Geometry check sheet. Reference: the model listing, model coordinates, mm. Give positions to 0.01 mm unless a question says otherwise; leave off trailing zeros. Loops run counter-clockwise (first coordinate to the right, second up) from the corner with the lowest first, then second, coordinate; pieces in that order, holes last.
1. Go/stop test with flat-tipped pins: pin 1 Ø1 at (y, z) = (-52, 1.5) entering from +X; pin 2 Ø3 at (y, z) = (-34, 9) entering from +X. Record where each tip stops, or that it passes through.
2. Cross-section at D-D, the plane y = -17. Record the cut outline in (x, z).
3. Cross-section at B-B, the plane x = -126.5. Record the cut outline in (y, z).
4. Release check for a two-part mould opening along Y. For faces 1 (the cylindrical face through (85.467, -33.361, 6.261)), 2 (the flat face through (-11, -32, 0)), 3 (the cylindrical face through (-153.58, -31.57, 6.26)) record: +Y half, -Y half, draft (parallel to the pull), parting line (faces both ways), or undercut.
5. Cross-section at A-A, the plane y = -28.5. Record the cut outline in (x, z).
6. Material ranges on L1, parallel to X at y = -32.5, z = 11.25; L2, parallel to X at y = -39, z = 11; L3, parallel to Y at x = -142.5, z = 6.5, recorded low to high.
from build123d import *

# Parameters (mm, degrees)
SKETCH1_R           = 20.32
BOSS_EXTRUDE1_DEPTH = 12.7


with BuildPart() as part:
    # Sketch1 → Boss-Extrude1 (new body)
    with BuildSketch(Plane.XY):
        with BuildLine():
            Line((37.409275597, 7.872494736), (-133.278879175, -7.060783805))
            ThreePointArc((-133.278879175, -7.060783805), (-158.678879175, -32.460783805), (-133.278879175, -57.860783805))
            Line((-133.278879175, -57.860783805), (37.409275597, -72.794062346))
            Line((37.409275597, -72.794062346), (44.521120825, -73.41626818))
            ThreePointArc((44.521120825, -73.41626818), (85.476605199, -32.460783805), (44.521120825, 8.49470057))
            Line((44.521120825, 8.49470057), (37.409275597, 7.872494736))
        make_face()
        with Locations((-133.278879175, -32.460783805)):
            Circle(SKETCH1_R, mode=Mode.SUBTRACT)
        with Locations((44.521120825, -32.460783805)):
            Circle(SKETCH1_R, mode=Mode.SUBTRACT)
    extrude(amount=BOSS_EXTRUDE1_DEPTH)


solid = part.part
Result:
1. pin 1: stops at x = 80.78
1. pin 2: stops at x = 85.48
2. outline: (-153.43, 0) - (-146.46, 0) - (-146.46, 12.7) - (-153.43, 12.7) - close; (-120.09, 0) - (31.34, 0) - (31.34, 12.7) - (-120.09, 12.7) - close; (57.71, 0) - (82.45, 0) - (82.45, 12.7) - (57.71, 12.7) - close
3. outline: (-58.45, 0) - (-51.62, 0) - (-51.62, 12.7) - (-58.45, 12.7) - close; (-13.3, 0) - (-6.47, 0) - (-6.47, 12.7) - (-13.3, 12.7) - close
4. face 1: parting line
4. face 2: draft
4. face 3: undercut
5. outline: (-158.37, 0) - (-153.21, 0) - (-153.21, 12.7) - (-158.37, 12.7) - close; (-113.35, 0) - (24.59, 0) - (24.59, 12.7) - (-113.35, 12.7) - close; (64.45, 0) - (85.28, 0) - (85.28, 12.7) - (64.45, 12.7) - close
6. L1: x = -158.68 to -153.6, -112.96 to 24.2, 64.84 to 85.48
6. L2: x = -157.82 to -152.52, -114.04 to 25.28, 63.76 to 84.95
6. L3: y = -56.13 to -50.57, -14.35 to -8.79
